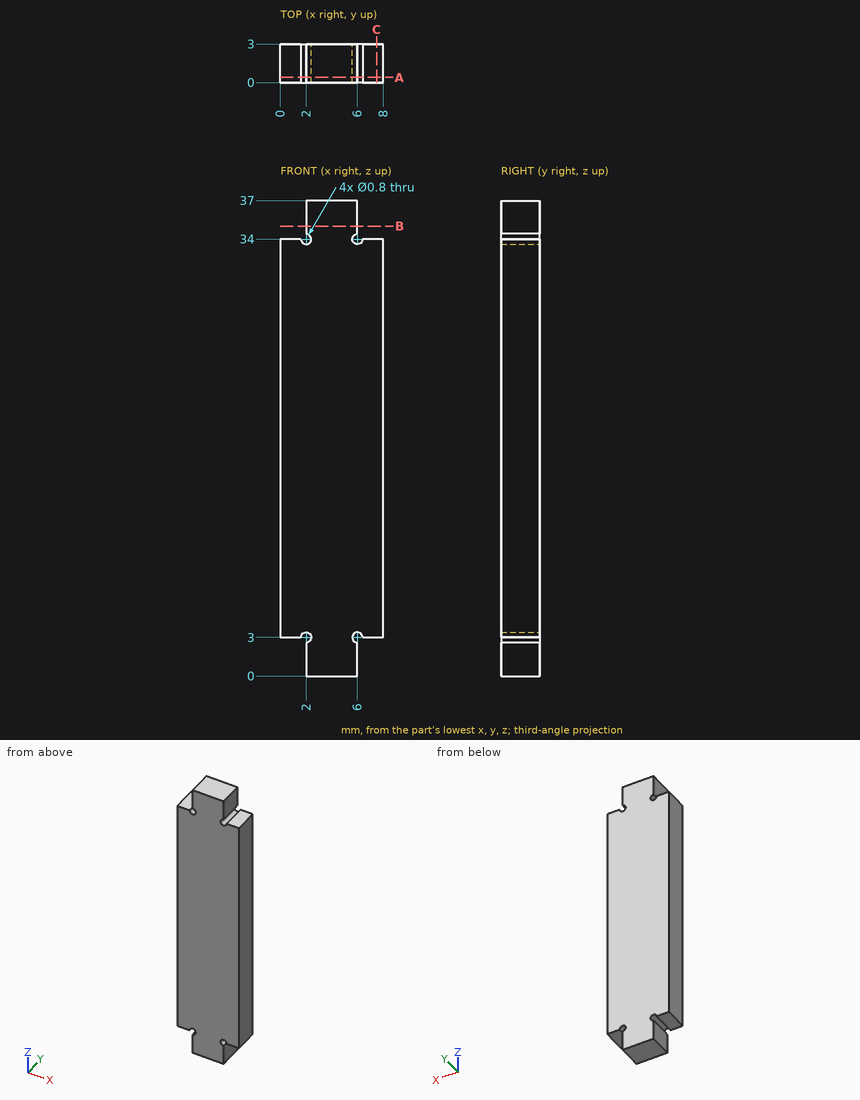
Input: dimensioned drawing with shaded views. Units: mm. Origin: part minimum x, y, z. Give positions to 0.01 mm unless a question says otherwise; leave off trailing zeros. Write each loop counter-clockwise with the first axis right and the second up, starting at its lowest first coordinate (ties: lowest second). Pieces come first, ordered by that corner, then holes.
Q1. Section A-A, the plane y = 0.4. Output: boundary loops of the cut face in (x, z), plus the area to 3 significant figures.
Q2. First-contact query: P1, Ø0.8, axis at y = 2, z = 35.5, coming from the +X side; P2, Ø0.8, axis at x = 1, y = 1.5, coming from the +Z side; P3, Ø0.5, axis at x = 7.5, y = 2, coming from the -Z side. Flat tips, straight axial feed; report the tip coordinate or a pass-through.
Q3. Section B-B, the plane z = 35. Output: boundary loops of the cut face in (x, y), plus the area to 3 significant figures.
Q4. Material intervals for probe 1 along Z at (x, y) = (7.75, 1.3); probe 2 along Z at (x, y) = (6.25, 2.85), sorted ascending.
Q5. Section C-C, the plane x = 7.5. Output: boundary loops of the cut face in (y, z), plus the area to 3 significant figures.
Filled in:
1. outline: (0, 3) - (1.6, 3) arc R0.4 cw (long way) to (2, 2.6) - (2, 0) - (6, 0) - (6, 2.6) arc R0.4 cw (long way) to (6.4, 3) - (8, 3) - (8, 34) - (6.4, 34) arc R0.4 cw (long way) to (6, 34.4) - (6, 37) - (2, 37) - (2, 34.4) arc R0.4 cw (long way) to (1.6, 34) - (0, 34) - close
1. area: 270 mm2
2. P1: stops at x = 6
2. P2: stops at z = 34
2. P3: stops at z = 3
3. outline: (2, 0) - (6, 0) - (6, 3) - (2, 3) - close
3. area: 12.0 mm2
4. probe 1: z = 3 to 34
4. probe 2: z = 3.31 to 33.69
5. outline: (0, 3) - (3, 3) - (3, 34) - (0, 34) - close
5. area: 93.0 mm2
